Input: part model. Units: mm. Frame: model coordinates. Face numbers are marked on the shaded views. Give positions to 0.01 mm unless a question says otherwise; leave off trailing zeros. Order: outer loops, then holes, each group sorted by start corner. A loop starts at its lowest first (then second) coordinate and runs counter-clockwise, first axis right, second up. Notation, with made-up numbers: (2, 49) - (57, 49) arc R34 ccw to (57, 84) - close; hole circle Ø1 at (52, 17). An arc over 180 degrees is marked (long way). Use a Markdown table: item, result.
Autodesk Inventor part; units mm, degrees
ref_plane "YZ Plane" through (0, 0, 0) normal (1, 0, 0) x (0, 1, 0)
ref_plane "XZ Plane" through (0, 0, 0) normal (0, 1, 0) x (-1, 0, 0)
ref_plane "XY Plane" through (0, 0, 0) normal (0, 0, 1) x (1, 0, 0)
sketch "Sketch1" plane through (0, 0, 0) normal (0, 1, 0) x (-1, 0, 0)
  circle A0 centre (0, 0) radius 135
  circle A1 centre (0, 0) radius 110
  dimension "d0" = 270
  dimension "d1" = 220
extrude "Extrusion1" add sketch "Sketch1" along normal blind 20
sketch "Sketch2" plane through (0, 0, 0) normal (0, 0, 1) x (1, 0, 0)
  circle A0 centre (0, 23) radius 18
  line L0 (135, 0) -> (-135, 0)
  point P0 (0, 0)
  dimension "d4" = 36
  dimension "d5" = 23
extrude "Extrusion2" cut sketch "Sketch2" against normal through all
sketch "Sketch3" plane through (0, 20, 0) normal (0, 1, 0) x (1, 0, 0)
  circle A0 centre (0, 0) radius 127.5
  circle A1 centre (-127.5, 0) radius 2
  circle A2 centre (-103.1497, -74.9426) radius 2
  circle A3 centre (-39.3997, -121.2597) radius 2
  circle A4 centre (39.3997, -121.2597) radius 2
  circle A5 centre (103.1497, -74.9426) radius 2
  circle A6 centre (127.5, 0) radius 2
  circle A7 centre (103.1497, 74.9426) radius 2
  circle A8 centre (39.3997, 121.2597) radius 2
  circle A9 centre (-39.3997, 121.2597) radius 2
  circle A10 centre (-103.1497, 74.9426) radius 2
  dimension "d8" = 255
  dimension "d9" = 4
  dimension "d12" = 360
hole "Hole1" at (103.1497, 20, 74.9426) at (127.5, 20, 0) at (103.1497, 20, -74.9426) at (39.3997, 20, -121.2597) at (-39.3997, 20, -121.2597) at (-103.1497, 20, -74.9426) at (-127.5, 20, 0) at (-103.1497, 20, 74.9426) at (-39.3997, 20, 121.2597) at (39.3997, 20, 121.2597) direction (0, -1, 0) diameter 5 end through all
sketch "Sketch4" plane through (0, 0, 0) normal (0, -1, 0) x (1, 0, 0)
  circle A0 centre (0, 0) radius 131.5
  circle A1 centre (0, 0) radius 135
  dimension "d21" = 263
extrude "Extrusion3" add sketch "Sketch4" along normal blind 2.5
properties part number "Cylinder Bottom"
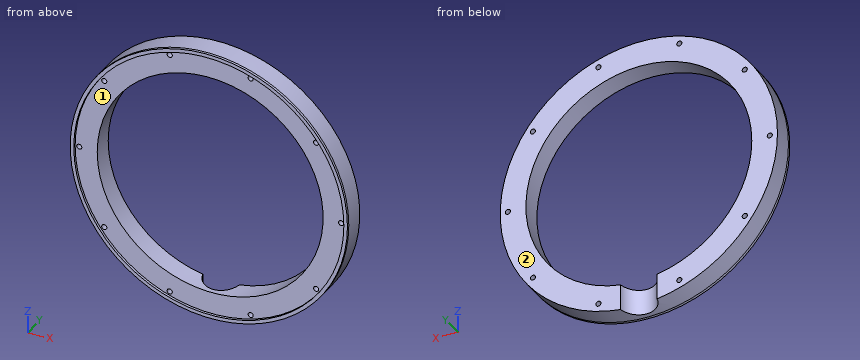
1. Pin query (flat end, axial travel): pin 1 (6 mm diameter, centred on x = 39.4, z = 121.26, fed in from -Y); pin 2 (8 mm diameter, centred on y = 1, z = -22.5, fed in from -X); pin 3 (3 mm diameter, centred on x = 68, y = 16, fed in from -Z); pin 4 (4.5 mm diameter, centred on x = -39.4, z = -121.26, fed in from +Y). Return the tip coordinate at first contact, or that it passes through.
Response:
| item | result |
|---|---|
| pin 1 | stops at y = 0 |
| pin 2 | stops at x = -133.73 |
| pin 3 | stops at z = -117.49 |
| pin 4 | passes through |
2. Section query C-C (y = 14). State how many separate pieces and enclosed holes the cut face has, then the cut area to 3 significant figures.
Response:
| item | result |
|---|---|
| separate pieces | 1 |
| enclosed holes | 10 |
| area | 18,300 mm^2 |
3. Section query B-B (z = 67). Return loops of the section in (x, y).
Response:
| item | result |
|---|---|
| outline | (-117.2, -2.5) - (-113.15, -2.5) - (-113.15, 0) - (-87.24, 0) - (-87.24, 20) - (-117.2, 20) - close; (87.24, 0) - (113.15, 0) - (113.15, -2.5) - (117.2, -2.5) - (117.2, 20) - (87.24, 20) - close |
4. Mould query, pull axis X, two halves, no side actions, for the marked faces 1 and 2. Classes: pulls with the +X half, pulls with the -X half, needs draft (parallel to the pull), parting line crosses it, or undercut.
Response:
| item | result |
|---|---|
| face 1 | undercut |
| face 2 | needs draft |
5. Section query A-A (x = 0). Return loops of the section in (y, z).
Response:
| item | result |
|---|---|
| outline | (-2.5, -135) - (5, -135) - (5, -110) - (0, -110) - (0, -131.5) - (-2.5, -131.5) - close; (-2.5, 131.5) - (0, 131.5) - (0, 110) - (20, 110) - (20, 135) - (-2.5, 135) - close |
6. Material intervals for line 1 along X through (y, z) = (9, 0); line 2 along Z through (x, y) = (0, -1.05); line 3 along X through (y, z) = (3.5, 3.5), sorted ascending.
Response:
| item | result |
|---|---|
| line 1 | x = -135 to -130, -125 to -110, 110 to 125, 130 to 135 |
| line 2 | z = -135 to -131.5, 131.5 to 135 |
| line 3 | x = -134.95 to -109.94, 109.94 to 134.95 |
